Could you check a few things on this drawing? It's one solid part, dimensions in mm from its lowest x, y, z. A direction names the side the tool comes from. Give positions to 0.01 mm unless a question says otherwise; leave off trailing zeros. Write each loop counter-clockwise with the first axis right and the second up, starting at its lowest first coordinate (ties: lowest second). Pieces come first, ordered by that corner, then holes.
1. If I drill on probe 1 along Y at (x, z) = (5, 1.15); probe 2 along Z at (x, y) = (14.45, 9.8); probe 3 along Z at (x, y) = (17.75, 2.75), over which ranges is the centre line in solid material (lowest first)?
2. Thinking about a two-plate mould opening in X: for the marked faces 1, 2 and 3, which applies, pulls with the +X half, pulls with the -X half, needs draft (parallel to the pull), parting line crosses it, or undercut?
3. Suppose I cut it at C-C (z = 12). Please give me the cut outline in (x, y), and give its area (3 significant figures).
4. Suppose I cut it at B-B (y = 17.5). Please give me the cut outline in (x, z), and give its area (3 significant figures).
5. On a 3-axis mill with a long thin cutter (end or side, diameter ignored), from which of +Z, -Z, +X, -X, +Y, -Y can I reach the whole of each face in a straight line? I mean the marked faces 4, 5 and 6. Say none if no direction works.
6. Suppose I cut it at A-A (x = 14.45). Please give me the cut outline in (y, z).
7. I'm going to push flat-ended pins straight in: pin 1 (2.5 mm diameter, centred on x = 19.5, y = 17, fed in from +Z); pin 2 (10 mm diameter, centred on x = 10.5, z = 15, fed in from -Y); pin 3 (12 mm diameter, centred on x = 12, z = 13, fed in from +Y). Where does each tip first touch, or does it pass through?
8. Suppose I cut it at D-D (x = 24.25). Please give me the cut outline in (y, z), and give its area (3 significant figures).
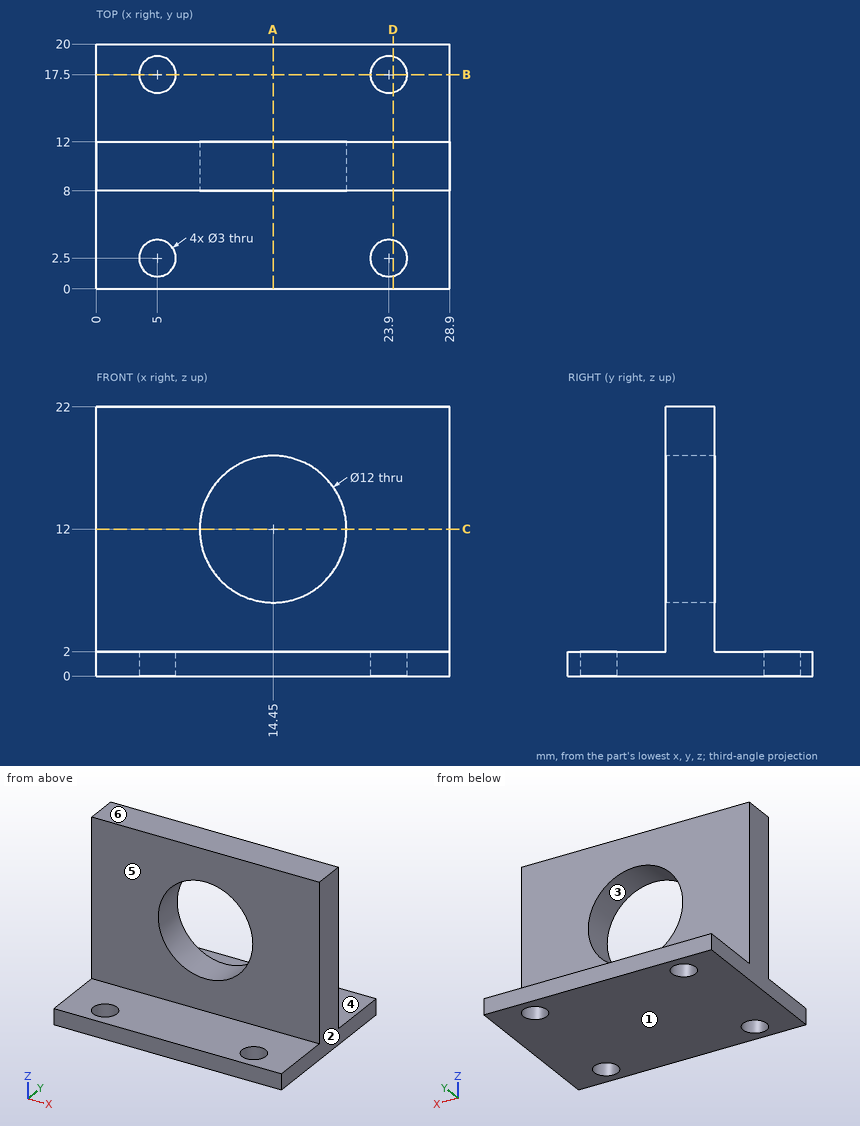
Checks:
1. probe 1: y = 0 to 1, 4 to 16, 19 to 20
1. probe 2: z = 0 to 6, 18 to 22
1. probe 3: z = 0 to 2
2. face 1: needs draft
2. face 2: pulls with the +X half
2. face 3: undercut
3. outline: (0, 8) - (8.45, 8) - (8.45, 12) - (0, 12) - close; (20.45, 8) - (28.9, 8) - (28.9, 12) - (20.45, 12) - close
3. area: 67.6 mm2
4. outline: (0, 0) - (3.5, 0) - (3.5, 2) - (0, 2) - close; (6.5, 0) - (22.4, 0) - (22.4, 2) - (6.5, 2) - close; (25.4, 0) - (28.9, 0) - (28.9, 2) - (25.4, 2) - close
4. area: 45.8 mm2
5. face 4: +Z, +X, -X, +Y
5. face 5: +Z, +X, -X, -Y
5. face 6: +Z, +X, -X, +Y, -Y
6. outline: (0, 0) - (20, 0) - (20, 2) - (12, 2) - (12, 6) - (8, 6) - (8, 2) - (0, 2) - close; (8, 18) - (12, 18) - (12, 22) - (8, 22) - close
7. pin 1: stops at z = 2
7. pin 2: stops at y = 8
7. pin 3: stops at y = 12
8. outline: (0, 0) - (1.04, 0) - (1.04, 2) - (0, 2) - close; (3.96, 0) - (16.04, 0) - (16.04, 2) - (12, 2) - (12, 22) - (8, 22) - (8, 2) - (3.96, 2) - close; (18.96, 0) - (20, 0) - (20, 2) - (18.96, 2) - close
8. area: 108 mm2
